Check sheet for the modelled part. Datum: model origin and axes. Units: mm. A direction names the side the tool comes from. Coordinates: 2 decimals unless noted, no trailing zeros. Write each loop counter-clockwise with the first axis right and the second up, starting at its lowest first coordinate (ties: lowest second). Pieces come first, ordered by that corner, then holes. Notation, with made-up numbers: (75, 21.25) - (92, 21.25) arc R28 cw to (92, 48.25) - close; hole circle Ø7 at (18.25, -18.5). An arc over 180 degrees is marked (long way). Answer as CSV lines item,"result". Start each with the question number.
from build123d import *

# Parameters (mm, degrees)
BOSS_EXTRUDE1_DEPTH = 10
SKETCH3_R           = 2.5
CUT_EXTRUDE1_DEPTH  = 10
BOSS_EXTRUDE2_DEPTH = 5
SKETCH9_W           = 6.522192951
SKETCH9_H           = 3.955645811
BOSS_EXTRUDE3_DEPTH = 10
CHAMFER1_SIZE       = 1
SKETCH12_R          = 2
CUT_EXTRUDE4_DEPTH  = 10


with BuildPart() as part:
    # Sketch1 → Boss-Extrude1 (new body)
    with BuildSketch(Plane(origin=(0, 0, 0), x_dir=(1, 0, 0), z_dir=(0, 1, 0))):
        with BuildLine():
            Line((52.5, 10), (30.923292192, 10))
            ThreePointArc((30.923292192, 10), (0, 32.5), (-30.923292192, 10))
            Line((-30.923292192, 10), (-52.5, 10))
            Line((-52.5, 10), (-52.5, 0))
            Line((-52.5, 0), (-30, 0))
            ThreePointArc((-30, 0), (0, 30), (30, 0))
            Line((30, 0), (52.5, 0))
            Line((52.5, 0), (52.5, 10))
        make_face()
    extrude(amount=BOSS_EXTRUDE1_DEPTH)

    # Sketch3 → Cut-Extrude1 (cut)
    with BuildSketch(Plane.XY):
        with Locations((-41.25, 5)):
            Circle(SKETCH3_R)
        with Locations((41.25, 5)):
            Circle(SKETCH3_R)
    extrude(amount=-CUT_EXTRUDE1_DEPTH, mode=Mode.SUBTRACT)

    # Sketch5 → Boss-Extrude2 (add)
    with BuildSketch(Plane(origin=(0, 0, 0), x_dir=(1, 0, 0), z_dir=(0, 1, 0))):
        with BuildLine():
            ThreePointArc((37.5, 0), (0, 37.5), (-37.5, 0))
            Line((-37.5, 0), (-32.5, 0))
            ThreePointArc((-32.5, 0), (0, 32.5), (32.5, 0))
            Line((32.5, 0), (37.5, 0))
        make_face()
    extrude(amount=BOSS_EXTRUDE2_DEPTH)

    # Sketch9 → Boss-Extrude3 (add)
    with BuildSketch(Plane.XZ):
        with Locations((31.545367723, -11.977822906)):
            Rectangle(SKETCH9_W, SKETCH9_H)
    extrude(amount=BOSS_EXTRUDE3_DEPTH)

    # Chamfer1
    chamfer1_edges = [part.edges().sort_by_distance(p)[0] for p in [
        (28.284271247, -10, -11.977822906),
        (34.806464198, -10, -11.977822906),
    ]]
    chamfer(chamfer1_edges, length=CHAMFER1_SIZE)

    # Sketch12 → Cut-Extrude4 (cut)
    with BuildSketch(Plane(origin=(0, 0, -13.955645811), x_dir=(-1, 0, 0), z_dir=(0, 0, -1))):
        with Locations((-31.545367723, -6)):
            Circle(SKETCH12_R)
    extrude(amount=-CUT_EXTRUDE4_DEPTH, mode=Mode.SUBTRACT)


solid = part.part
(1) Cross-section at B-B on x = 41.25. Record the boundary of the cut face in (y, z).
(2) Go/stop test with flat-tipped pins: P1, Ø3, axis at x = -45, y = 6, coming from the -Z side; P2, Ø2, axis at y = -5.5, z = -12.5, coming from the +X side; P3, Ø3, axis at y = -3.5, z = -12, coming from the -X side. Record where each tip stops, or that it passes through.
(3) Material ranges on probe 1 along Y at (x, z) = (-41.25, -5.5); probe 2 along X at (y, z) = (6.5, -1.5); probe 3 along Y at (x, z) = (-2, -34), recorded low to high. Write a range as from..to.
(4) Cross-section at C-C on z = -12.5. Record the boundary of the cut face in (x, y).
(5) Release check for a two-part mould opening along X. For faces 1 (the face through (38.6, 4.9, 0)), 2 (the face through (-0.66, 4.93, -29.993)), 3 (the face through (52.5, 5, -5)) record: pulls with the +X half, pulls with the -X half, needs draft (parallel to the pull), parting line crosses it, or undercut.
(6) Cross-section at D-D on z = -22. Record the boundary of the cut face in (x, y).
(7) Cross-section at A-A on y = 6.5. Record the boundary of the cut face in (x, z), plus the area to 3 significant figures.
(8) Tool access check on faces 4 (the face through (28.284, -4, -12)), 5 (the face through (44, 5, -10)), 6 (the face through (-3, 5, -33)), 7 (the face through (31.5, -3.8, -10)), 8 (the face through (34.806, -4, -12)). Record the directions out of +Z, -Z, +X, -X, +Y, -Y that give a thin tool (end or side, any length) a straight path to the whole face; none if there is none.
Checked values:
1,outline,"(0, -10) - (2.5, -10) - (2.5, 0) - (0, 0) - close; (7.5, -10) - (10, -10) - (10, 0) - (7.5, 0) - close"
2,P1,"z = -10"
2,P2,"x = 34.81"
2,P3,"x = 28.28"
3,probe 1,"0..2.5, 7.5..10"
3,probe 2,"-52.5..-43.25, -39.25..-29.96, 29.96..39.25, 43.25..52.5"
3,probe 3,"0..5"
4,outline,"(-35.36, 0) - (-27.27, 0) - (-27.27, 10) - (-30, 10) - (-30, 5) - (-35.36, 5) - close; (27.27, 0) - (28.28, 0) - (28.28, -9) - (29.28, -10) - (33.81, -10) - (34.81, -9) - (34.81, 0) - (35.36, 0) - (35.36, 5) - (30, 5) - (30, 10) - (27.27, 10) - close; hole circle Ø4 at (31.55, -6)"
5,face 1,"needs draft"
5,face 2,"undercut"
5,face 3,"pulls with the +X half"
6,outline,"(-30.37, 0) - (-20.4, 0) - (-20.4, 10) - (-23.92, 10) - (-23.92, 5) - (-30.37, 5) - close; (20.4, 0) - (30.37, 0) - (30.37, 5) - (23.92, 5) - (23.92, 10) - (20.4, 10) - close"
7,outline,"(-52.5, -10) - (-43.25, -10) - (-43.25, 0) - (-52.5, 0) - close; (-39.25, -10) - (-30.92, -10) arc R32.5 ccw to (30.92, -10) - (39.25, -10) - (39.25, 0) - (30, 0) arc R30 cw to (-30, 0) - (-39.25, 0) - close; (43.25, -10) - (52.5, -10) - (52.5, 0) - (43.25, 0) - close"
7,area,"576 mm^2"
8,face 4,"+Z, -Z, -X, -Y"
8,face 5,"-Z, +X, +Y"
8,face 6,"-Z, +Y"
8,face 7,"+Z, +X, -X, -Y"
8,face 8,"+Z, -Z, +X, -Y"
